Geometry: final body of the model. Coordinates: model frame, mm. A direction names the side the tool comes from. Give positions to 0.01 mm unless a question says otherwise; leave off trailing zeros. Order: outer loops, then holes, each group sorted by start corner. A loop starts at its lowest first (then second) coordinate and runs counter-clockwise, first axis right, second up. Notation, with made-up numbers: (49.5, -39.75) - (60.5, -39.75) arc R15 ccw to (60.5, -13.75) - close; hole circle Ø6 at (88, -33). An arc over 180 degrees is marked (long way). Put each result on its own line as item: value. Start each with the question number.
1. Set-up query: faces 4 (the flat face through (76.2, 11, -11)), 5 (the flat face through (4.696, 50.163, -0.444)), 6 (the flat face through (37.7, 27.881, 47.403)), 7 (the flat face through (71.5, -24.7, 43.67)), 8 (the flat face through (71.5, 24.7, -43.67)). Return all of +Z, -Z, +X, -X, +Y, -Y with unobstructed straight access to the full face (end or side cutting, diameter ignored); none if empty.
2. Section C-C on z = 0. Return the cut outline in (x, y) (3 decimals), plus the area to 3 significant figures.
3. Section B-B on y = -32. Return the cut outline in (x, z) (3 decimals), plus the area to 3 significant figures.
4. Section D-D on x = 39.5. Return the cut outline in (y, z), plus the area to 3 significant figures.
5. First-contact query: P1, Ø4, axis at x = 46.5, y = -10, coming from the -Z side; P2, Ø2, axis at x = 46, z = 39.5, coming from the +Y side; P3, Ø1.5, axis at x = 35, z = 49, coming from the +Y side. Flat tips, straight axial feed; report the tip coordinate or a pass-through.
6. Ray query, line 1 along X through (y, z) = (-17.5, 12.5); line 2 along Z through (x, y) = (193.5, 1); line 3 along X through (y, z) = (-2.5, 52.5). Return the intervals inside material, ascending. Write a range as from..to.
7. Section A-A on z = -16.5. Return the cut outline in (x, y) (3 decimals), plus the area to 3 significant figures.
8. Mould query, pull axis X, two halves, no side actions, for faces 1 (the flat face through (233.296, -50.163, 0.444)), 2 (the flat face through (267.1, 27.11, -47.85)), 3 (the flat face through (300.104, 50.163, -0.444)). Classes: pulls with the +X half, pulls with the -X half, needs draft (parallel to the pull), parting line crosses it, or undercut.
from build123d import *

# Parameters (mm, degrees)
BASE_EXTRUDE_DEPTH  = 76.2
CHAMFER1_SIZE       = 9.525
SKETCH2_R           = 12.691316964
BOSS_EXTRUDE1_DEPTH = 76.2


with BuildPart() as part:
    # Sketch1 → Base-Extrude (new body)
    with BuildSketch(Plane(origin=(0, 0, 0), x_dir=(0, 0, -1), z_dir=(1, 0, 0))):
        Polygon((63.5, 0), (31.75, 54.99261314), (-31.75, 54.99261314), (-63.5, 0), (-31.75, -54.99261314), (31.75, -54.99261314), align=None)
    extrude(amount=BASE_EXTRUDE_DEPTH)

    # Chamfer1
    chamfer1_edges = [part.edges().sort_by_distance(p)[0] for p in [
        (76.2, 54.99261314, 0),
        (76.2, 27.49630657, 47.625),
        (76.2, -27.49630657, 47.625),
        (76.2, -54.99261314, 0),
        (76.2, -27.49630657, -47.625),
        (0, -54.99261314, 0),
        (0, -27.49630657, 47.625),
        (0, 27.49630657, 47.625),
        (76.2, 27.49630657, -47.625),
        (0, 54.99261314, 0),
        (0, 27.49630657, -47.625),
        (0, -27.49630657, -47.625),
    ]]
    chamfer(chamfer1_edges, length=CHAMFER1_SIZE)

    # Sketch2 → Boss-Extrude1 (add)
    with BuildSketch(Plane(origin=(76.2, 0, 0), x_dir=(0, 0, -1), z_dir=(1, 0, 0))):
        with Locations(Location((0, 0, 0), (0, 0, 180))):
            Circle(SKETCH2_R)
    extrude(amount=BOSS_EXTRUDE1_DEPTH)

    # Mirror All1: part across plane


with BuildPart() as part_1:
    add(part.part)
    add(part.part.mirror(Plane(origin=(152.4, 0, 0), x_dir=(0, 0, 1), z_dir=(1, 0, 0))))


solid = part_1.part
Resolved:
1. face 4: none
1. face 5: +Z, -Z, -X, +Y
1. face 6: +Z, +X, -X, +Y
1. face 7: +Z, -Y
1. face 8: -Z, +Y
2. outline: (0, -45.468) - (9.525, -54.993) - (66.675, -54.993) - (76.2, -45.468) - (76.2, -12.691) - (228.6, -12.691) - (228.6, -45.468) - (238.125, -54.993) - (295.275, -54.993) - (304.8, -45.468) - (304.8, 45.468) - (295.275, 54.993) - (238.125, 54.993) - (228.6, 45.468) - (228.6, 12.691) - (76.2, 12.691) - (76.2, 45.468) - (66.675, 54.993) - (9.525, 54.993) - (0, 45.468) - close
2. area: 20,300 mm^2
3. outline: (0, -34.026) - (9.525, -45.025) - (66.675, -45.025) - (76.2, -34.026) - (76.2, 34.026) - (66.675, 45.025) - (9.525, 45.025) - (0, 34.026) - close; (228.6, -34.026) - (238.125, -45.025) - (295.275, -45.025) - (304.8, -34.026) - (304.8, 34.026) - (295.275, 45.025) - (238.125, 45.025) - (228.6, 34.026) - close
3. area: 13,300 mm^2
4. outline: (-54.99, -31.75) - (0, -63.5) - (54.99, -31.75) - (54.99, 31.75) - (0, 63.5) - (-54.99, 31.75) - close
4. area: 10,500 mm^2
5. P1: z = -58.88
5. P2: y = 43.3
5. P3: y = 26.41
6. line 1: 0..76.2, 228.6..304.8
6. line 2: -12.65..12.65
6. line 3: 1.25..74.95, 229.85..303.55
7. outline: (0, -45.468) - (9.525, -54.993) - (66.675, -54.993) - (76.2, -45.468) - (76.2, 45.468) - (66.675, 54.993) - (9.525, 54.993) - (0, 45.468) - close; (228.6, -45.468) - (238.125, -54.993) - (295.275, -54.993) - (304.8, -45.468) - (304.8, 45.468) - (295.275, 54.993) - (238.125, 54.993) - (228.6, 45.468) - close
7. area: 16,400 mm^2
8. face 1: undercut
8. face 2: needs draft
8. face 3: pulls with the +X half
